```python
from build123d import *

# Parameters (mm, degrees)
F0_W     = 76.2
F0_H     = 19.05
F1_DEPTH = 20.828
F3_DEPTH = 76.2
F4_R     = 4.699
F5_DEPTH = 41.276


# Not quite as in the source:
# - ends of sketch curves that miss each other by under 0.0002 mm in the source are joined


with BuildPart() as f1:
    # F0 (on Front) → F1 (new body)
    with BuildSketch(Plane.XZ):
        Polygon((-23.8125, 0), (-52.3875009418, 0), (-52.3875009418, 28.575), (-76.2000009418, 28.575), (-76.2000009418, 0), (-76.2, -3.175), (0, -3.175), (0, 0), (0, 28.575), (-23.8125, 28.575), align=None)
        with Locations((-38.1, -12.7)):
            Rectangle(F0_W, F0_H)
    extrude(amount=F1_DEPTH)

    # F2 (on Right) → F3 (join)
    with BuildSketch(Plane.YZ):
        Polygon((0, -22.225), (-20.828, -22.225), (-65.278, -22.225), (-65.278, -41.275), (29.972, -41.275), (29.972, -22.225), align=None)
    extrude(amount=-F3_DEPTH)

    # F4 (on Top) → F5 (cut, through all)
    with BuildSketch(Plane.XY):
        with Locations((-12.7, 17.272)):
            Circle(F4_R)
        with Locations((-12.7, -52.578)):
            Circle(F4_R)
        with Locations((-63.5, -52.578)):
            Circle(F4_R)
        with Locations((-63.5, 17.272)):
            Circle(F4_R)
    extrude(amount=-F5_DEPTH, mode=Mode.SUBTRACT)


solid = f1.part
```
Check sheet for the modelled part. Datum: model origin and axes. Units: mm. A direction names the side the tool comes from. Coordinates: 2 decimals unless noted, no trailing zeros. Loops run counter-clockwise (first coordinate to the right, second up) from the corner with the lowest first, then second, coordinate; pieces in that order, holes last. Notation, with made-up numbers: M -26.5,69.25 L 14.5,69.25 A16 ccw 14.5,92.25 Z; hole C -31,89.5 d2. An arc over 180 degrees is marked long. Answer as a JSON object with one key per item and string values.
1. Depth check by flat-ended pin: P1, Ø3, axis at x = -58.5, z = 5, coming from the +Y side; P2, Ø3, axis at x = -37, z = -4, coming from the -Y side; P3, Ø12, axis at x = -63.5, y = -52.578, coming from the +Z side (3 decimals). Enter the tip coordinate at first touch or a pass-through.
Outcome:
{"P1": "y = 0", "P2": "y = -20.83", "P3": "z = -22.225"}
2. Sectioned sample at D-D on z = -30. Record the cut outline in (x, y), and give its area (3 significant figures).
Outcome:
{"outline": "M -76.2,-65.28 L 0,-65.28 L 0,29.97 L -76.2,29.97 Z; hole C -63.5,-52.58 d9.4; hole C -63.5,17.27 d9.4; hole C -12.7,-52.58 d9.4; hole C -12.7,17.27 d9.4", "area": "6,980 mm²"}
3. Sectioned sample at C-C on y = 14.5. Record the cut outline in (x, z) (3 decimals), and give its area (3 significant figures).
Outcome:
{"outline": "M -76.2,-41.275 L -67.294,-41.275 L -67.294,-22.225 L -76.2,-22.225 Z; M -59.706,-41.275 L -16.494,-41.275 L -16.494,-22.225 L -59.706,-22.225 Z; M -8.906,-41.275 L 0,-41.275 L 0,-22.225 L -8.906,-22.225 Z", "area": "1,160 mm²"}
4. Scan lines: L1, parallel to X at y = 17.5, z = -38; L2, parallel to Y at x = -63.5, z = -33.5; L3, parallel to Y at x = -63, z = -35. Record each from-to range of solid material in increasing order. Write a range as from..to.
Outcome:
{"L1": "-76.2..-68.19, -58.81..-17.39, -8.01..0", "L2": "-65.28..-57.28, -47.88..12.57, 21.97..29.97", "L3": "-65.28..-57.25, -47.91..12.6, 21.94..29.97"}
5. Sectioned sample at A-A on x = -63.5. Record the cut outline in (y, z) (3 decimals), and give its area (3 significant figures).
Outcome:
{"outline": "M -65.278,-41.275 L -57.277,-41.275 L -57.277,-22.225 L -65.278,-22.225 Z; M -47.879,-41.275 L 12.573,-41.275 L 12.573,-22.225 L 0,-22.225 L 0,28.575 L -20.828,28.575 L -20.828,-22.225 L -47.879,-22.225 Z; M 21.971,-41.275 L 29.972,-41.275 L 29.972,-22.225 L 21.971,-22.225 Z", "area": "2,510 mm²"}
6. Release check for a two-part mould opening along Y. For faces 6 (the cylindrical face through (-16.16, -49.4, -31.62)), 7 (the flat face through (-38, 29.972, -32)), 8 (the flat face through (-64, -10, 28.575)), 9 (the cylindrical face through (-13.31, 21.93, -31.62)) record: pulls with the +Y half, pulls with the -Y half, needs draft (parallel to the pull), parting line crosses it, or undercut.
Outcome:
{"face 6": "undercut", "face 7": "pulls with the +Y half", "face 8": "needs draft", "face 9": "undercut"}
7. Access from +Z, -Z, +X, -X, +Y, -Y to the whole of each face (thin tool, end or side, straight path). Record for faces 1 (the flat face through (-38, -65.278, -32)), 2 (the cylindrical face through (-59.018, -51.167, -31.617)), 3 (the flat face through (-38, -43, -22.225)), 4 (the flat face through (-38, 15, -22.225)), 5 (the flat face through (-52.388, -10, 14)).
Outcome:
{"face 1": "+Z, -Z, +X, -X, -Y", "face 2": "+Z, -Z", "face 3": "+Z, +X, -X, -Y", "face 4": "+Z, +X, -X, +Y", "face 5": "+Z, +Y, -Y"}
8. Sectioned sample at B-B on y = -7.5. Record the cut outline in (x, z) (1 decimal), and give its area (3 significant figures).
Outcome:
{"outline": "M -76.2,-41.3 L 0,-41.3 L 0,28.6 L -23.8,28.6 L -23.8,0 L -52.4,0 L -52.4,28.6 L -76.2,28.6 L -76.2,0 L -76.2,-3.2 Z", "area": "4,510 mm²"}
